CAD build for the part. Positions are in the model's coordinates, mm. Coordinates: 2 decimals unless noted, no trailing zeros. Write each loop counter-clockwise with the first axis right and the second up, starting at its lowest first coordinate (ties: lowest second). Pieces come first, ordered by that corner, then holes. Notation, with made-up numbers: (-19, 48) - (20, 48) arc R14 cw to (20, 66) - close; hole circle Ø10 at (18.25, 47). An arc over 180 degrees is marked (long way). Answer in a Markdown table with one row per item. Add a question column.
Q1. Drill centre lines: line 1 along Z through (x, y) = (-89, -192); line 2 along X through (y, z) = (-1319, -1); line 3 along X through (y, z) = (-821, 2). Where is each one in solid material? Low to high. Write a range as from..to.
Q2. Band-saw the part on B-B (x = -83.5). List the corners of the cut face in (y, z), and give its area (3 significant figures).
Q3. Pin check, flat tip, straight feed: pin 1 (3 mm diameter, centred on x = -69.5, y = -388, fed in from +Z). Stop position of the tip, or through.
Q4. Band-saw the part on A-A (y = -392). List the corners of the cut face in (x, z).
```python
from build123d import *

# Parameters (mm, degrees)
F1_DEPTH = 1400


# Not quite as in the source:
# - ends of sketch curves that miss each other by under 0.0002 mm in the source are joined


with BuildPart() as f1:
    # F0 (on Front) → F1 (new body)
    with BuildSketch(Plane.XZ):
        with BuildLine():
            ThreePointArc((-102.8194582262, -1.753334156), (-102.8759917705, -1.6691495307), (-102.9300627594, -1.5833624634))
            ThreePointArc((-102.9300627594, -1.5833624634), (-105.3062912412, 3.621474375), (-106.1115923498, 9.2861260008))
            Line((-106.1115923498, 9.2861260008), (-136.111652, 9.288465))
            Line((-136.111652, 9.288465), (-136.111652, -30.711535))
            Line((-136.111652, -30.711535), (-16.111652, -30.711535))
            Line((-16.111652, -30.711535), (-16.111652, 9.288465))
            Line((-16.111652, 9.288465), (-46.111705, 9.288465))
            ThreePointArc((-46.111705, 9.288465), (-46.9260256459, 3.5907327912), (-49.3292641557, -1.6391538962))
            ThreePointArc((-49.3292641557, -1.6391538962), (-49.348739835, -1.6694199812), (-49.3685261016, -1.6994839384))
            ThreePointArc((-49.3685261016, -1.6994839384), (-50.6166534947, -2.8386108222), (-52.2530199988, -3.2601991421))
            Line((-52.2530199988, -3.2601991421), (-52.3114330011, -3.260199))
            Line((-52.3114330011, -3.260199), (-99.942409, -3.260199))
            ThreePointArc((-99.942409, -3.260199), (-101.566297382, -2.8606806598), (-102.8194582262, -1.753334156))
        make_face()
    extrude(amount=F1_DEPTH)


solid = f1.part
```
Checked values:
| question | item | result |
|---|---|---|
| 1 | line 1 | z = -30.71..-3.26 |
| 1 | line 2 | x = -136.11..-103.29, -48.93..-16.11 |
| 1 | line 3 | x = -136.11..-104.76, -47.47..-16.11 |
| 2 | outline | (-1400, -30.71) - (0, -30.71) - (0, -3.26) - (-1400, -3.26) - close |
| 2 | area | 38,400 mm² |
| 3 | pin 1 | stops at z = -3.26 |
| 4 | outline | (-136.11, -30.71) - (-16.11, -30.71) - (-16.11, 9.29) - (-46.11, 9.29) arc R20 cw to (-49.33, -1.64) arc R3.5 cw to (-49.37, -1.7) arc R3.5 cw to (-52.25, -3.26) - (-52.31, -3.26) - (-99.94, -3.26) arc R3.5 cw to (-102.93, -1.58) arc R20 cw to (-106.11, 9.29) - (-136.11, 9.29) - close |
